Part print with two shaded views. Sizes in mm from the minimum x, y, z corner. A direction names the side the tool comes from. Coordinates: 2 decimals unless noted, no trailing zeros. Loops run counter-clockwise (first coordinate to the right, second up) from the corner with the lowest first, then second, coordinate; pieces in that order, holes last.
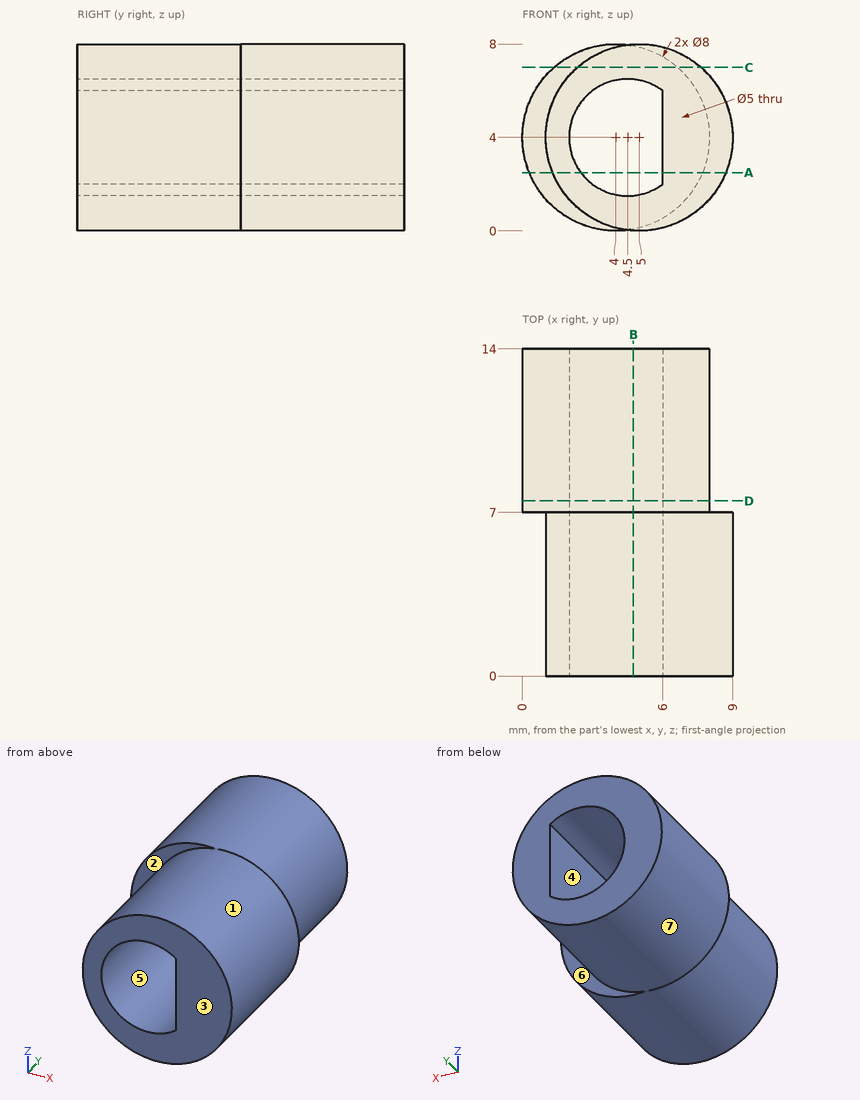
Q1. Mould opens along Z. For the marked faces 5, 6 and 7 say: +Z half, -Z half, draft (parallel to the pull), parting line (faces both ways), or undercut.
Answers:
face 5: undercut
face 6: draft
face 7: parting line
Q2. Slice it at A-A (z = 2.5). List the corners of the cut face in (x, y), and give its area (3 significant figures).
Answers:
outline: (0.29, 7) - (1.29, 7) - (1.29, 0) - (2.5, 0) - (2.5, 14) - (0.29, 14) - close; (6, 0) - (8.71, 0) - (8.71, 7) - (7.71, 7) - (7.71, 14) - (6, 14) - close
area: 54.8 mm2
Q3. Flat gauge pin, fed straight in: P1, Ø3, axis at y = 5, z = 4.5, coming from the -X side. Where does the tip first touch, or does it go through?
Answers:
P1: stops at x = 1
Q4. Slice it at B-B (x = 4.75). List the corners of the cut face in (y, z).
Answers:
outline: (0, 0.01) - (7, 0.01) - (7, 0.07) - (14, 0.07) - (14, 1.51) - (0, 1.51) - close; (0, 6.49) - (14, 6.49) - (14, 7.93) - (7, 7.93) - (7, 7.99) - (0, 7.99) - close
Q5. Which spindle directions (+Z, -Z, +X, -X, +Y, -Y) get a long thin tool onto all of the face, cutting with end or side? Do the marked faces 1, 2, 3 and 4. Say none if no direction does.
Answers:
face 1: -Y
face 2: -X, -Y
face 3: +Z, -Z, +X, -X, -Y
face 4: +Y, -Y
Q6. Slice it at D-D (y = 7.5). List the corners of the cut face in (x, z).
Answers:
outline: circle Ø8 at (4, 4); hole (6, 2) - (6, 6) arc R2.5 ccw (long way) to start
Q7. Drill centre lines: line 1 (Y direction, x = 8.5, z = 4.25); line 2 (X direction, y = 12.5, z = 5); line 3 (Z direction, x = 4.5, y = 6.75). Where is each one in solid material? Low to high.
Answers:
line 1: y = 0 to 7
line 2: x = 0.13 to 2.21, 6 to 7.87
line 3: z = 0.03 to 1.5, 6.5 to 7.97
Q8. Slice it at C-C (z = 7). List the corners of the cut face in (x, y), and give its area (3 significant figures).
Answers:
outline: (1.35, 7) - (2.35, 7) - (2.35, 0) - (7.65, 0) - (7.65, 7) - (6.65, 7) - (6.65, 14) - (1.35, 14) - close
area: 74.1 mm2
